Here's how the part is built. I have some questions about the finished solid (model axes, mm). A direction names the side the tool comes from. Coordinates: 2 decimals unless noted, no trailing zeros. Write each loop counter-clockwise with the first axis right and the second up, starting at its lowest first coordinate (ties: lowest second). Pieces come first, ordered by that corner, then holes. Notation, with made-up numbers: M 39,19.5 L 76,19.5 A28 cw 76,54.5 Z; hole C 1,73.25 d2. An arc over 180 degrees is marked long. Use a Markdown table: item, result.
Autodesk Inventor part; units mm, degrees
ref_plane "YZ Plane" through (0, 0, 0) normal (1, 0, 0) x (0, 1, 0)
ref_plane "XZ Plane" through (0, 0, 0) normal (0, 1, 0) x (-1, 0, 0)
ref_plane "XY Plane" through (0, 0, 0) normal (0, 0, 1) x (1, 0, 0)
sketch "Sketch1" plane through (0, 0, 0) normal (0, 1, 0) x (-1, 0, 0)
  line L0 (0, 0) -> (-22.86, 0)
  line L1 (-22.86, 0) -> (-22.86, -22.86)
  line L2 (-22.86, -22.86) -> (0, -22.86)
  line L3 (0, -22.86) -> (0, 0)
  line L4 (-22.86, -22.86) -> (-19.304, -22.86)
  line L5 (-19.304, -22.86) -> (-19.304, -19.304) construction
  line L6 (-19.304, -19.304) -> (-22.86, -19.304) construction
  line L7 (-22.86, -19.304) -> (-22.86, -22.86)
  line L8 (0, -22.86) -> (-3.556, -22.86)
  line L9 (-3.556, -22.86) -> (-3.556, -19.304) construction
  line L10 (-3.556, -19.304) -> (0, -19.304) construction
  line L11 (0, -19.304) -> (0, -22.86)
  line L12 (0, 0) -> (-3.556, 0)
  line L13 (-3.556, 0) -> (-3.556, -3.556) construction
  line L14 (-3.556, -3.556) -> (0, -3.556) construction
  line L15 (0, -3.556) -> (0, 0)
  line L16 (-22.86, 0) -> (-19.304, 0)
  line L17 (-19.304, 0) -> (-19.304, -3.556) construction
  line L18 (-19.304, -3.556) -> (-22.86, -3.556) construction
  line L19 (-22.86, -3.556) -> (-22.86, 0)
  circle A0 centre (-3.556, -19.304) radius 2.032
  circle A1 centre (-19.304, -19.304) radius 2.032
  circle A2 centre (-19.304, -3.556) radius 2.032
  circle A3 centre (-3.556, -3.556) radius 2.032
  line L20 (3.57, -26.43) -> (-26.43, -26.43)
  line L21 (-26.43, -26.43) -> (-26.43, 3.57)
  line L22 (-26.43, 3.57) -> (3.57, 3.57)
  line L23 (3.57, 3.57) -> (3.57, -26.43)
  line L24 (0, 0) -> (-6.5, 0)
  line L25 (-6.5, 0) -> (-6.5, -6.5)
  line L26 (-6.5, -6.5) -> (0, -6.5)
  line L27 (0, -6.5) -> (0, 0)
  line L28 (0, -22.86) -> (-6.5, -22.86)
  line L29 (-6.5, -22.86) -> (-6.5, -16.36)
  line L30 (-6.5, -16.36) -> (0, -16.36)
  line L31 (0, -16.36) -> (0, -22.86)
  line L32 (-22.86, -22.86) -> (-16.36, -22.86)
  line L33 (-16.36, -22.86) -> (-16.36, -16.36)
  line L34 (-16.36, -16.36) -> (-22.86, -16.36)
  line L35 (-22.86, -16.36) -> (-22.86, -22.86)
  line L36 (-22.86, 0) -> (-16.36, 0)
  line L37 (-16.36, 0) -> (-16.36, -6.5)
  line L38 (-16.36, -6.5) -> (-22.86, -6.5)
  line L39 (-22.86, -6.5) -> (-22.86, 0)
  line L40 (-26.43, 3.57) -> (-49.205, 3.57)
  line L41 (-49.205, 3.57) -> (-49.205, -26.43)
  line L42 (-49.205, -26.43) -> (-26.43, -26.43)
  line L43 (-26.43, -26.43) -> (-26.43, 3.57)
  circle A4 centre (-11.43, -11.43) radius 5
  point P0 (0, -16.36)
  point P1 (0, -6.5)
  dimension "d2" = 22.86
  dimension "d3" = 22.86
  dimension "d4" = 3.556
  dimension "d5" = 3.556
  dimension "d6" = 3.556
  dimension "d7" = 3.556
  dimension "d8" = 3.556
  dimension "d9" = 3.556
  dimension "d10" = 3.556
  dimension "d11" = 3.556
  dimension "d12" = 4.064
  dimension "d13" = 4.064
  dimension "d14" = 4.064
  dimension "d15" = 4.064
  dimension "d16" = 30
  dimension "d17" = 30
  dimension "d18" = 3.57
  dimension "d19" = 3.57
  dimension "d20" = 6.5
  dimension "d21" = 6.5
  dimension "d22" = 6.5
  dimension "d23" = 6.5
  dimension "d24" = 6.5
  dimension "d25" = 6.5
  dimension "d26" = 6.5
  dimension "d31" = 10
  dimension "d32" = 15
  dimension "d33" = 15
  dimension "d34" = 37.775
extrude "Extrusion1" add sketch "Sketch1" along normal blind 7 contours L3 L26 L25 L0 | L37 L38 L1 L0 | L3 L2 L29 L30 | L34 L33 L2 L1 | L20 L21 L22 L23 | L42 L41 L40 L21
fillet "Fillet1" radius 2 4 edges at (6.5, 3.5, -16.36) (16.36, 3.5, -16.36) (16.36, 3.5, -6.5) (6.5, 3.5, -6.5)
sketch "Sketch4" plane through (49.205, 0, 3.57) normal (1, 0, 0) x (0, 0, -1)
  line L0 (-10, 13.5061) -> (40, 13.5061)
  line L1 (40, 13.5061) -> (40, -6.4939)
  line L2 (40, -6.4939) -> (-10, -6.4939)
  line L3 (-10, -6.4939) -> (-10, 13.5061)
  line L4 (-10, 13.5061) -> (40, -6.4939) construction
  line L5 (40, 13.5061) -> (-10, -6.4939) construction
  line L6 (30, 0) -> (30, 7)
  line L7 (15, 3.5061) -> (35, 3.5061)
  circle A0 centre (35, 3.5061) radius 1.625
  circle A1 centre (-5, 3.5061) radius 1.625
  line L8 (-10, 0) -> (40, 0)
  line L9 (40, 0) -> (40, 13.5061)
  line L10 (40, 13.5061) -> (-10, 13.5061)
  line L11 (-10, 13.5061) -> (-10, 0)
  line L12 (-10, -6.4939) -> (0, -6.4939)
  line L13 (0, -6.4939) -> (0, 0)
  line L14 (0, 0) -> (-10, 0)
  line L15 (-10, 0) -> (-10, -6.4939)
  line L16 (40, -6.4939) -> (30, -6.4939)
  line L17 (30, -6.4939) -> (30, 0)
  line L18 (30, 0) -> (40, 0)
  line L19 (40, 0) -> (40, -6.4939)
  line L20 (40, 13.5061) -> (20, 13.5061)
  line L21 (20, 13.5061) -> (20, 6.753)
  line L22 (20, 6.753) -> (40, 6.753)
  line L23 (40, 6.753) -> (40, 13.5061)
  line L24 (0, 7) -> (30, 7)
  line L25 (-10, 13.5061) -> (10, 13.5061)
  line L26 (10, 13.5061) -> (10, 7)
  line L27 (10, 7) -> (-10, 7)
  line L28 (-10, 7) -> (-10, 13.5061)
  point P0 (3.57, 0)
  point P1 (40, -3.247)
  point P2 (-10, -3.247)
  point P3 (-10, 10.253)
  point P4 (10, 10.253)
  point P5 (40, 10.1296)
  point P6 (20, 13.5061)
  point P7 (10, 13.5061)
  point P8 (-10, 7)
  point P9 (40, 6.753)
  dimension "d46" = 50
  dimension "d47" = 20
  dimension "d48" = 15
  dimension "d49" = 10
  dimension "d56" = 20
  dimension "d57" = 20
  dimension "d58" = 3.25
  dimension "d59" = 3.25
  dimension "d66" = 10
  dimension "d67" = 20
  dimension "d68" = 20
extrude "Extrusion4" add sketch "Sketch4" against normal blind 5 contours L0 L21 L24 L26 | L27 L24 L21 L22 L6 L8 L3 | L8 L13 L2 L3 | L8 L17 L2 L13 | L1 L8 L6 L22 | L8 L1 L2 L17
fillet "Fillet2" radius 5 2 edges at (-3.57, 3.5, -26.43) (-3.57, 3.5, 3.57)
chamfer "Chamfer1" distance 10 angle 45 2 edges at (46.705, -6.4939, 13.57) (46.705, -6.4939, -36.43)
sketch "Sketch5" plane through (0, 0, 0) normal (0, -1, 0) x (1, 0, 0)
  line L0 (1.43, 3.57) -> (44.205, 3.57)
  line L1 (-3.57, -26.43) -> (22.8175, -26.43) construction
  line L2 (22.8175, -26.43) -> (22.8175, 3.57) construction
  line L3 (22.8175, 3.57) -> (-3.57, 3.57) construction
  line L4 (-3.57, 3.57) -> (-3.57, -26.43) construction
  line L5 (0, -22.86) -> (22.8175, -22.86) construction
  line L6 (22.8175, -22.86) -> (22.8175, 0) construction
  line L7 (22.8175, 0) -> (0, 0) construction
  line L8 (0, 0) -> (0, -22.86) construction
  circle A0 centre (11.43, -11.43) radius 11.43 construction
  line L9 (0, -6.5) -> (0, -16.36)
  line L10 (16.36, 0) -> (6.5, 0)
  line L11 (6.5, -22.86) -> (16.36, -22.86)
sketch "Sketch6" plane through (0, 0, 0) normal (0, -1, 0) x (1, 0, 0)
  line L0 (0, -6.5) -> (0, -16.36)
  line L1 (16.36, 0) -> (6.5, 0)
  line L2 (22.86, -16.36) -> (22.86, -6.5)
  line L3 (6.5, -22.86) -> (16.36, -22.86)
  circle A0 centre (11.43, -11.43) radius 11.43
  point P0 (0, 0)
properties part number "as5600mount"
1. Suppose I cut it at B-B on z = -31.43. Write out the boundary of the cut face in (x, y) (3 decimals).
Answers follow:
| item | result |
|---|---|
| outline | M 44.205,-1.494 L 49.205,-1.494 L 49.205,1.881 L 44.205,1.881 Z; M 44.205,5.131 L 49.205,5.131 L 49.205,6.753 L 44.205,6.753 Z |
2. Suppose I cut it at C-C on x = 40. Write out the boundary of the cut face in (y, z), and give its area (3 significant figures).
Answers follow:
| item | result |
|---|---|
| outline | M 0,-26.43 L 7,-26.43 L 7,3.57 L 0,3.57 Z |
| area | 210 mm2 |
3. Which directions (+Z, -Z, +X, -X, +Y, -Y) give clear straight access to the entire face, cutting with the end or side of a thin tool? Please do faces 1 (the face through (-2.07, 3.55, -25)), 2 (the face through (23, 3, 3.57)), 3 (the face through (47, 10, -16.43)), 4 (the face through (47, -6.494, -12)), 5 (the face through (22.86, 3, -11)).
Answers follow:
| item | result |
|---|---|
| face 1 | -Z, -X, +Y, -Y |
| face 2 | +Z, -X, +Y, -Y |
| face 3 | -Z, +X, -X, +Y |
| face 4 | +Z, -Z, +X, -X, -Y |
| face 5 | +Y, -Y |
4. Will these pins go through, and if not, where does the flat tip stop? pin 1 Ø3.5 at (x, y) = (3, 2) entering from +Z; pin 2 Ø8 at (x, y) = (24.5, 0) entering from -Z; pin 3 Ø5.5 at (x, z) = (19.304, -3.556) entering from -Y.
Answers follow:
| item | result |
|---|---|
| pin 1 | stops at z = 3.57 |
| pin 2 | stops at z = -26.43 |
| pin 3 | stops at y = 0 |
5. Suppose I cut it at A-A on x = 15. Write out the boundary of the cut face in (y, z).
Answers follow:
| item | result |
|---|---|
| outline | M 0,-26.43 L 7,-26.43 L 7,-22.86 L 0,-22.86 Z; M 0,0 L 7,0 L 7,3.57 L 0,3.57 Z |
6. We'd pull the mould along Z, two halves only. Please class faces 6 (the face through (-2.14, 3.55, 2.07)), 7 (the face through (23.2, 7, -10.6)), 8 (the face through (5.17, 3.45, -2.32)): +Z half, -Z half, draft (parallel to the pull), parting line (faces both ways), or undercut.
Answers follow:
| item | result |
|---|---|
| face 6 | +Z half |
| face 7 | draft |
| face 8 | undercut |
7. Suppose I cut it at D-D on y = -5. Write out the boundary of the cut face in (x, z) (3 decimals).
Answers follow:
| item | result |
|---|---|
| outline | M 44.205,-27.924 L 49.205,-27.924 L 49.205,5.064 L 44.205,5.064 Z |
8. I need wall thicknesses on probe 1 along Z at (x, y) = (13, 0.5); probe 2 along Z at (x, y) = (4.5, 2); probe 3 along X at (y, z) = (-3.5, -23) (3 decimals). Which ranges of each line are inside material? Lowest first, please.
Answers follow:
| item | result |
|---|---|
| probe 1 | z = -26.43 to -22.86, 0 to 3.57 |
| probe 2 | z = -26.43 to -21.1, -17.5 to -16.36, -6.5 to -5.36, -1.76 to 3.57 |
| probe 3 | x = 44.205 to 49.205 |
